from build123d import *

# Parameters (mm, degrees)
SKETCH1_R          = 2.6
SKETCH1_R_2        = 3.1
BASE_FLANGE1_DEPTH = 3
FILLET_10_MM_R     = 10
FILLET1_R          = 7
FILLET2_START      = -4
FILLET2_DEPTH      = 5
FILLET2_START_2    = -3
FILLET2_2_DEPTH    = 3


with BuildPart() as part:
    # Base-Flange1: sheet metal written as solids
    # Sketch1 → Base-Flange1 (new body)
    with BuildSketch(Plane.XY):
        Polygon((-31, -5.857930586), (-10, -5.857930586), (-10, 0.142069414), (10, 0.142069414), (10, -5.857930586), (31, -5.857930586), (31, -45.857930586), (5, -65.857930586), (-5, -65.857930586), (-31, -45.857930586), align=None)
        with Locations((25, -12.857930586)):
            Circle(SKETCH1_R, mode=Mode.SUBTRACT)
        with Locations((-25, -12.857930586)):
            Circle(SKETCH1_R, mode=Mode.SUBTRACT)
        with Locations((0, -9.857930586)):
            Circle(SKETCH1_R_2, mode=Mode.SUBTRACT)
        with Locations((5, -32.957930586)):
            Circle(SKETCH1_R, mode=Mode.SUBTRACT)
        with Locations((-5, -32.957930586)):
            Circle(SKETCH1_R, mode=Mode.SUBTRACT)
        with BuildLine():
            Line((-2.6, -55.457930586), (-2.6, -50.257930586))
            ThreePointArc((-2.6, -50.257930586), (0, -47.657930586), (2.6, -50.257930586))
            Line((2.6, -50.257930586), (2.6, -55.457930586))
            ThreePointArc((2.6, -55.457930586), (0, -58.057930586), (-2.6, -55.457930586))
        make_face(mode=Mode.SUBTRACT)
    extrude(amount=-BASE_FLANGE1_DEPTH)

    # fillet 10 mm
    fillet_10_mm_edges = [part.edges().sort_by_distance(p)[0] for p in [
        (31, -45.857930586, -1.5),
        (5, -65.857930586, -1.5),
        (-5, -65.857930586, -1.5),
        (-31, -45.857930586, -1.5),
    ]]
    fillet(fillet_10_mm_edges, radius=FILLET_10_MM_R)

    # Fillet1
    fillet1_edges = [part.edges().sort_by_distance(p)[0] for p in [
        (31, -5.857930586, -1.5),
        (-31, -5.857930586, -1.5),
    ]]
    fillet(fillet1_edges, radius=FILLET1_R)

    # Fillet2: read off the stored shape, not the designer's step
    # Fillet2 outline → Fillet2 (cut)
    with BuildSketch(Plane.XY.offset(FILLET2_START)):
        with BuildLine():
            Line((-10, 0.142069414), (-10, -2.857930586))
            ThreePointArc((-10, -2.857930586), (-9.121320344, -0.736610242), (-7, 0.142069414))
            Line((-7, 0.142069414), (-10, 0.142069414))
        make_face()
        with BuildLine():
            Line((10, 0.142069414), (7, 0.142069414))
            ThreePointArc((7, 0.142069414), (9.121320344, -0.736610242), (10, -2.857930586))
            Line((10, -2.857930586), (10, 0.142069414))
        make_face()
    extrude(amount=FILLET2_DEPTH, mode=Mode.SUBTRACT)

    # Fillet2 2 outline → Fillet2 2 (add)
    with BuildSketch(Plane.XY.offset(FILLET2_START_2)):
        with BuildLine():
            Line((-10, -5.857930586), (-10, -2.857930586))
            ThreePointArc((-10, -2.857930586), (-10.878679656, -4.97925093), (-13, -5.857930586))
            Line((-13, -5.857930586), (-10, -5.857930586))
        make_face()
        with BuildLine():
            ThreePointArc((13, -5.857930586), (10.878679656, -4.97925093), (10, -2.857930586))
            Line((10, -2.857930586), (10, -5.857930586))
            Line((10, -5.857930586), (13, -5.857930586))
        make_face()
    extrude(amount=FILLET2_2_DEPTH)


solid = part.part
Build history of the part. All positions in model axes, mm. A direction names the side the tool comes from. Coordinates: 2 decimals unless noted, no trailing zeros. Order: outer loops, then holes, each group sorted by start corner. A loop starts at its lowest first (then second) coordinate and runs counter-clockwise, first axis right, second up. Notation, with made-up numbers: (76.5, 63.25) - (120.5, 63.25) arc R23 ccw to (120.5, 100.25) - close; hole circle Ø3 at (-5, 43). An arc over 180 degrees is marked (long way). Put each result on its own line as item: value.
1. Saw through at B-B (x = -25.5). Write the cut outline in (y, z), and give its area (3 significant figures).
Answer sheet:
outline: (-50.09, -3) - (-15.41, -3) - (-15.41, 0) - (-50.09, 0) - close; (-10.31, -3) - (-6.02, -3) - (-6.02, 0) - (-10.31, 0) - close
area: 117 mm^2
2. Pull direction Y, two halves, no side cores. Call faces 1 (the face through (-2.6, -53, -1)), 2 (the face through (17.53, -56.22, -1.48)), 3 (the face through (0.057, -58.057, -1.479)), 4 (the face through (28.895, -7.854, -1.521)): pulls with the +Y half, pulls with the -Y half, needs draft (parallel to the pull), parting line crosses it, or undercut.
Answer sheet:
face 1: undercut
face 2: pulls with the -Y half
face 3: undercut
face 4: pulls with the +Y half
3. Saw through at D-D (x = 25). Write the cut outline in (y, z).
Answer sheet:
outline: (-50.47, -3) - (-15.46, -3) - (-15.46, 0) - (-50.47, 0) - close; (-10.26, -3) - (-5.93, -3) - (-5.93, 0) - (-10.26, 0) - close
4. Saw through at C-C (z = -0.6). Write the cut outline in (x, y), and give its area (3 significant figures).
Answer sheet:
outline: (-31, -40.93) arc R10 ccw to (-27.1, -48.86) - (-7.7, -63.78) arc R10 ccw to (-1.6, -65.86) - (1.6, -65.86) arc R10 ccw to (7.7, -63.78) - (27.1, -48.86) arc R10 ccw to (31, -40.93) - (31, -12.86) arc R7 ccw to (24, -5.86) - (13, -5.86) arc R3 cw to (10, -2.86) arc R3 ccw to (7, 0.14) - (-7, 0.14) arc R3 ccw to (-10, -2.86) arc R3 cw to (-13, -5.86) - (-24, -5.86) arc R7 ccw to (-31, -12.86) - close; hole circle Ø5.2 at (-25, -12.86); hole circle Ø5.2 at (-5, -32.96); hole circle Ø6.2 at (0, -9.86); hole (-2.6, -55.46) arc R2.6 ccw to (2.6, -55.46) - (2.6, -50.26) arc R2.6 ccw to (-2.6, -50.26) - close; hole circle Ø5.2 at (5, -32.96); hole circle Ø5.2 at (25, -12.86)
area: 3,130 mm^2
5. Tool access for faces 5 (the face through (18, -5.858, -1)), 6 (the face through (0, -65.858, -1)), 7 (the face through (-0.06, -47.66, -1.48)): list every direction of +Z, -Z, +X, -X, +Y, -Y with a clear straight run to the whole face (end or side of a thin tool).
Answer sheet:
face 5: +Z, -Z, +X, +Y
face 6: +Z, -Z, +X, -X, -Y
face 7: +Z, -Z
6. Saw through at A-A (x = 0). Write the cut outline in (y, z), and give its area (3 significant figures).
Answer sheet:
outline: (-65.86, -3) - (-58.06, -3) - (-58.06, 0) - (-65.86, 0) - close; (-47.66, -3) - (-12.96, -3) - (-12.96, 0) - (-47.66, 0) - close; (-6.76, -3) - (0.14, -3) - (0.14, 0) - (-6.76, 0) - close
area: 148 mm^2
7. Probe line 1 along X through (y, z) = (-3, -0.6); line 2 along Y through (x, z) = (-5, -1.5); line 3 along X through (y, z) = (-31, -2.6). List the from-to ranges inside material, lowest first. Write a range as [from, to].
Answer sheet:
line 1: x = [-10, 10]
line 2: y = [-65.26, -35.56], [-30.36, 0.14]
line 3: x = [-31, -6.71], [-3.29, 3.29], [6.71, 31]
8. Drop flat-ended pins along their axis: P1, Ø1, axis at x = 6.5, y = -51, coming from the +Z side; P2, Ø3, axis at x = 25, y = -12.86, coming from the -Z side (3 decimals); P3, Ø0.9, axis at y = -52.5, z = -1, coming from the +X side; P4, Ø1, axis at x = 20.5, z = -2.5, coming from the +Y side. Give the stop position or say it passes through.
Answer sheet:
P1: stops at z = 0
P2: passes through
P3: stops at x = 22.95
P4: stops at y = -5.86
